```python
from build123d import *

# Parameters (mm, degrees)
SKETCH_1_W          = 50
SKETCH_1_H          = 44
SKETCH_1_R          = 1.953838975
SKETCH_1_R_2        = 13
EXTRUDE_1_DEPTH     = 3
SKETCH_2_W          = 3
SKETCH_2_H          = 44
EXTRUDE_2_DEPTH     = 50
SKETCH_3_R          = 1.5
CUT_EXTRUDE_1_DEPTH = 77.111759932
SKETCH_4_R          = 12.2
CUT_EXTRUDE_2_DEPTH = 1
CHAMFER_1_SIZE      = 0.3


with BuildPart() as part:
    # 草图1 → 凸台-拉伸1 (new body)
    with BuildSketch(Plane(origin=(0, 0, 0), x_dir=(1, 0, 0), z_dir=(0, 1, 0))):
        Rectangle(SKETCH_1_W, SKETCH_1_H)
        with Locations(Location((0, 17.096091033, 0), (0, 0, 270))):
            Circle(SKETCH_1_R, mode=Mode.SUBTRACT)
        with Locations(Location((17.096091033, 0, 0), (0, 0, 270))):
            Circle(SKETCH_1_R, mode=Mode.SUBTRACT)
        with Locations(Location((0, -17.096091033, 0), (0, 0, 270))):
            Circle(SKETCH_1_R, mode=Mode.SUBTRACT)
        with Locations(Location((-17.096091033, 0, 0), (0, 0, 270))):
            Circle(SKETCH_1_R, mode=Mode.SUBTRACT)
        with Locations(Location((0, 0, 0), (0, 0, 270))):
            Circle(SKETCH_1_R_2, mode=Mode.SUBTRACT)
    extrude(amount=EXTRUDE_1_DEPTH)

    # 草图2 → 凸台-拉伸2 (add)
    with BuildSketch(Plane(origin=(0, 3, 0), x_dir=(1, 0, 0), z_dir=(0, 1, 0))):
        with Locations((-23.5, 0)):
            Rectangle(SKETCH_2_W, SKETCH_2_H)
        with Locations((23.5, 0)):
            Rectangle(SKETCH_2_W, SKETCH_2_H)
    extrude(amount=EXTRUDE_2_DEPTH)

    # 草图3 → 切除-拉伸1 (cut, through all)
    with BuildSketch(Plane.ZY.offset(25)):
        with Locations((0, 46)):
            Circle(SKETCH_3_R)
        with Locations((8, 38)):
            Circle(SKETCH_3_R)
        with Locations((0, 30)):
            Circle(SKETCH_3_R)
        with Locations((-8, 38)):
            Circle(SKETCH_3_R)
    extrude(amount=-CUT_EXTRUDE_1_DEPTH, mode=Mode.SUBTRACT)

    # 草图4 → 切除-拉伸2 (cut)
    with BuildSketch(Plane(origin=(25, 0, 0), x_dir=(0, 0, -1), z_dir=(1, 0, 0))):
        with Locations((0, 38)):
            Circle(SKETCH_4_R)
    cut_extrude_2 = extrude(amount=-CUT_EXTRUDE_2_DEPTH, mode=Mode.SUBTRACT)

    # 镜向1: 切除-拉伸2 across plane
    add(cut_extrude_2.mirror(Plane(origin=(0, 0, 0), x_dir=(0, 0, 1), z_dir=(1, 0, 0))), mode=Mode.SUBTRACT)

    # 倒角1
    chamfer_1_edges = [part.edges().sort_by_distance(p)[0] for p in [
        (-25, 38, 12.2),
        (0, 0, -13),
        (-25, 53, 0),
        (-23.5, 53, 22),
        (-22, 53, 0),
        (-23.5, 53, -22),
        (25, 53, 0),
        (23.5, 53, -22),
        (22, 53, 0),
        (23.5, 53, 22),
        (25, 0, 0),
        (-25, 0, 0),
        (25, 38, 12.2),
    ]]
    chamfer(chamfer_1_edges, length=CHAMFER_1_SIZE)


solid = part.part
```
CAD build for the part. Positions are in the model's coordinates, mm. A direction names the side the tool comes from. Coordinates: 2 decimals unless noted, no trailing zeros. Order: outer loops, then holes, each group sorted by start corner. A loop starts at its lowest first (then second) coordinate and runs counter-clockwise, first axis right, second up. Notation, with made-up numbers: M -36.5,35.5 L 13.5,35.5 A19 ccw 13.5,66.5 Z; hole C 27.25,12 d10. An arc over 180 degrees is marked long. Answer as CSV lines item,"result".
1) Flat gauge pins, fed straight in: P1, Ø12, axis at y = 36.5, z = 0, coming from the +X side; P2, Ø10, axis at x = -9.5, z = -9.5, coming from the +Y side; P3, Ø5, axis at y = 30, z = 0, coming from the -X side. Where does each tip first touch, or does it go through?
Verdict:
P1,"x = 24"
P2,"y = 3"
P3,"x = -24"
2) Cut at A-A (x = 0). List the corners of the cut face in (y, z).
Verdict:
outline,"M 0,-22 L 3,-22 L 3,-19.05 L 0,-19.05 Z; M 0,-15.14 L 3,-15.14 L 3,-13 L 0.3,-13 L 0,-13.3 Z; M 0,13.3 L 0.3,13 L 3,13 L 3,15.14 L 0,15.14 Z; M 0,19.05 L 3,19.05 L 3,22 L 0,22 Z"
3) 3-axis set-ups, long thin cutter, end or side, ignore diameter. For faces 5 (the flat face through (-10, 3, 9)), 6 (the cylindrical face through (-24.355, 48.287, -6.559)), 7 (the cylindrical face through (15.189, 1.479, -0.424)), 8 (the cylindrical face through (24.355, 48.287, -6.559)): which of +Z, -Z, +X, -X, +Y, -Y reach the whole face in a straight line?
Verdict:
face 5,"+Z, -Z, +Y"
face 6,"-X"
face 7,"+Y, -Y"
face 8,"+X"
4) Cut at B-B (y = 6). List the corners of the cut face in (x, z), then the cut area to 3 significant figures.
Verdict:
outline,"M -25,-22 L -22,-22 L -22,22 L -25,22 Z; M 22,-22 L 25,-22 L 25,22 L 22,22 Z"
area,"264 mm2"
5) Mould opens along Y. For faces 1 (the flat face through (-25, 20, 0)), 2 (the flat face through (-0.3, 0, -15)), 3 (the cylindrical face through (22.986, 36.536, -8.325)), 4 (the flat face through (-24, 53, 0)) say: released by +Y, released by -Y, zero draft, split by the parting line, or undercut.
Verdict:
face 1,"zero draft"
face 2,"released by -Y"
face 3,"undercut"
face 4,"released by +Y"
6) Cut at C-C (z = -14). List the corners of the cut face in (x, y), then the cut area to 3 significant figures.
Verdict:
outline,"M -25,0.3 L -24.7,0 L 24.7,0 L 25,0.3 L 25,52.7 L 24.7,53 L 22.3,53 L 22,52.7 L 22,3 L -22,3 L -22,52.7 L -22.3,53 L -24.7,53 L -25,52.7 Z"
area,"450 mm2"
7) Cut at D-D (x = -21). List the corners of the cut face in (y, z).
Verdict:
outline,"M 0,-22 L 3,-22 L 3,22 L 0,22 Z"
8) Drill centre lines: L1, parallel to Y at x = 22.85, z = 0; L2, parallel to X at y = 1.9, z = 0; L3, parallel to X at y = 34, z = -17.5. Where is each one in solid material? Low to high. Write a range as from..to.
Verdict:
L1,"0..28.5, 31.5..44.5, 47.5..53"
L2,"-25..-19.05, -15.14..-13, 13..15.14, 19.05..25"
L3,"-25..-22, 22..25"
